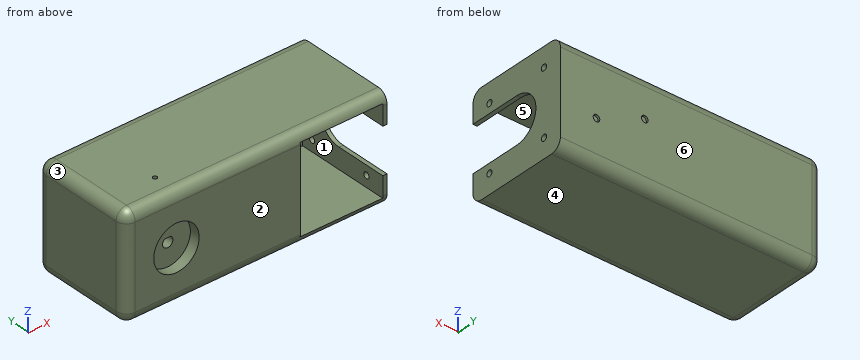
from build123d import *

# Parameters (mm, degrees)
F0_W           = 127
F0_H           = 50
F1_DEPTH       = 50
F3_DEPTH       = 42
F4_R           = 11
F5_DEPTH       = 5
F7_DEPTH       = 15
F8_T2_ANGLE    = 343.7894292622
F9_R           = 5
F12_W          = 40
F12_H          = 42
F13_DEPTH      = 46
F14_R          = 1.6
F15_DEPTH      = 1
F16_R          = 1
F17_DEPTH      = 2
F17_DEPTH_BACK = 1.03
F18_DEPTH      = 25
F19_DEPTH      = 2
F20_DEPTH      = 25


# Not quite as in the source:
# - a fillet or chamfer that OpenCascade refuses, or shapes differently, is made with other operations: its cross-section is extruded or revolved along the edge and cut away or added


with BuildPart() as f1:
    # F0 (on Front) → F1 (new body)
    with BuildSketch(Plane.XZ):
        Rectangle(F0_W, F0_H)
    extrude(amount=F1_DEPTH)

    # F2 (on face) → F3 (cut)
    with BuildSketch(Plane.YZ.offset(63.5)):
        Polygon((-41.7573593129, 21), (-46, 16.7573593129), (-46, -16.7573593129), (-41.7573593129, -21), (-8.2426406871, -21), (-4, -16.7573593129), (-4, 16.7573593129), (-8.2426406871, 21), align=None)
    extrude(amount=-F3_DEPTH, mode=Mode.SUBTRACT)

    # F4 (on face) → F5 (cut)
    with BuildSketch(Plane.XZ.offset(50)):
        with Locations((-38.5, 0)):
            Circle(F4_R)
    extrude(amount=-F5_DEPTH, mode=Mode.SUBTRACT)

    # F6 (on face) → F7 (cut)
    with BuildSketch(Plane.XZ.offset(45)):
        with BuildLine():
            Line((-37, 2), (-40, 2))
            ThreePointArc((-40, 2), (-38.5, -2.5), (-37, 2))
        make_face()
    extrude(amount=-F7_DEPTH, mode=Mode.SUBTRACT)

    # F8: fillet of radius 0.5 on 1 edges, made by hand

    # F8_s1 → F8_t2 (revolve)
    with BuildSketch(Plane(origin=(-37.7346622942, 0, -5.3739891953), x_dir=(0, 1, 0), z_dir=(0.9900106558, 0, 0.1409925581))):
        with BuildLine():
            ThreePointArc((-30.5, 7.9282134883), (-30.1464466094, 7.7817668789), (-30, 7.4282134883))
            Line((-30, 7.4282134883), (-30, 7.9282134883))
            Line((-30, 7.9282134883), (-30.5, 7.9282134883))
        make_face()
    revolve(axis=Axis((-38.5, -30, 0), (0, -1, 0)), revolution_arc=F8_T2_ANGLE)

    # F9
    f9_edges = [f1.edges().sort_by_distance(p)[0] for p in [
        (0, -50, 25),
        (0, -50, -25),
        (0, 0, 25),
        (0, 0, -25),
        (-63.5, -25, 25),
        (-63.5, -25, -25),
        (-63.5, 0, 0),
        (-63.5, -50, 0),
    ]]
    fillet(f9_edges, radius=F9_R)

    # F12 (on face) → F13 (cut)
    with BuildSketch(Plane.XZ.offset(50)):
        with Locations((41.5, 0)):
            Rectangle(F12_W, F12_H)
    extrude(amount=-F13_DEPTH, mode=Mode.SUBTRACT)

    # F14 (on face) → F15 (cut)
    with BuildSketch(Plane(origin=(0, 0, 0), x_dir=(-1, 0, 0), z_dir=(0, 1, 0))):
        with Locations((-46.0031795697, -4.1205275279)):
            Circle(F14_R)
        with Locations((-22.6282365388, 5.5031795697)):
            Circle(F14_R)
    extrude(amount=-F15_DEPTH, mode=Mode.SUBTRACT)

    # F16 (on face) → F17 (cut, two sides)
    with BuildSketch(Plane(origin=(0, 0, 2), x_dir=(1, 0, 0), z_dir=(0, 0, -1))) as f17_sk:
        Polygon((-36.5, 38.9047005384), (-38.5, 40.0594010768), (-40.5, 38.9047005384), (-40.5, 36.5952994616), (-38.5, 35.4405989232), (-36.5, 36.5952994616), align=None)
        with Locations((-38.5, 37.75)):
            Circle(F16_R, mode=Mode.SUBTRACT)
    extrude(amount=-F17_DEPTH, mode=Mode.SUBTRACT)
    extrude(f17_sk.sketch, amount=F17_DEPTH_BACK, mode=Mode.SUBTRACT)

    # F18 (cut): a face of the model
    f18_faces = [f1.faces().sort_by_distance(p)[0] for p in [
        (-38.5, -37.75, 2),
    ]]
    extrude(f18_faces, amount=-F18_DEPTH, mode=Mode.SUBTRACT)

    # F10 (on face) → F19 (join)
    with BuildSketch(Plane.YZ.offset(63.5)):
        Polygon((-46, 16.7573593129), (-46, -16.7573593129), (-41.7573593129, -21), (-8.2426406871, -21), (-4, -16.7573593129), (-4, 16.7573593129), (-8.2426406871, 21), (-16.9, 21), (-33.1, 21), (-41.7573593129, 21), align=None)
        with BuildLine():
            Line((-10.9, -15.6), (-39.1, -15.6))
            ThreePointArc((-39.1, -15.6), (-41.6606601718, -16.6606601718), (-40.6, -14.1))
            Line((-40.6, -14.1), (-40.6, 14.1))
            ThreePointArc((-40.6, 14.1), (-41.6606601718, 16.6606601718), (-39.1, 15.6))
            Line((-39.1, 15.6), (-10.9, 15.6))
            ThreePointArc((-10.9, 15.6), (-9.4, 17.1), (-7.9, 15.6))
            ThreePointArc((-7.9, 15.6), (-8.3393398282, 14.5393398282), (-9.4, 14.1))
            Line((-9.4, 14.1), (-9.4, -14.1))
            ThreePointArc((-9.4, -14.1), (-8.3393398282, -14.5393398282), (-7.9, -15.6))
            ThreePointArc((-7.9, -15.6), (-9.4, -17.1), (-10.9, -15.6))
        make_face(mode=Mode.SUBTRACT)
        with BuildLine():
            ThreePointArc((-40.6, -14.1), (-39.5393398282, -14.5393398282), (-39.1, -15.6))
            Line((-39.1, -15.6), (-10.9, -15.6))
            ThreePointArc((-10.9, -15.6), (-10.4606601718, -14.5393398282), (-9.4, -14.1))
            Line((-9.4, -14.1), (-9.4, 14.1))
            ThreePointArc((-9.4, 14.1), (-10.4606601718, 14.5393398282), (-10.9, 15.6))
            Line((-10.9, 15.6), (-39.1, 15.6))
            ThreePointArc((-39.1, 15.6), (-39.5393398282, 14.5393398282), (-40.6, 14.1))
            Line((-40.6, 14.1), (-40.6, -14.1))
        make_face()
    extrude(amount=-F19_DEPTH)

    # F11 (on face) → F20 (cut)
    with BuildSketch(Plane.YZ.offset(63.5)):
        with BuildLine():
            Line((-50, -11), (-25, -11))
            ThreePointArc((-25, -11), (-14, 0), (-25, 11))
            Line((-25, 11), (-50, 11))
            Line((-50, 11), (-50, -11))
        make_face()
    extrude(amount=-F20_DEPTH, mode=Mode.SUBTRACT)


solid = f1.part
Check sheet for the modelled part. Datum: model origin and axes. Units: mm. Face numbers are marked on the shaded views. A direction names the side the tool comes from. Give positions to 0.01 mm unless a question says otherwise; leave off trailing zeros. Loops run counter-clockwise (first coordinate to the right, second up) from the corner with the lowest first, then second, coordinate; pieces in that order, holes last. Notation, with made-up numbers: M 35,22 L 94,22 A23 cw 94,30 Z; hole C -29.5,22 d1. An arc over 180 degrees is marked long. Answer as a JSON object with one key per item and string values. Group by question number.
Q1. Material ranges on line 1 along X through (y, z) = (-32, -1.5); line 2 along X through (y, z) = (-7, 12.5); line 3 along Y through (x, z) = (62.7, -15.6), recorded low to high. Write a range as [from, to].
Q2. Cross-section at D-D on z = -9.5. Record the cut outline in (x, y), then the cut area to 3 significant figures.
Q3. Go/stop test with flat-tipped pins: P1, Ø1.8, axis at x = -38.5, y = -37.75, coming from the +Z side; P2, Ø17.5, axis at x = -38.5, z = 0, coming from the -Y side; P3, Ø1.9, axis at x = 46, z = -4.12, coming from the -Y side. Record where each tip stops, or that it passes through.
Q4. Release check for a two-part mould opening along Z. For the marked faces 1, 2, 3 and 4 record: released by +Z, released by -Z, zero draft, split by the parting line, or undercut.
Q5. Cross-section at A-A on x = 42. Record the cut outline in (y, z), then the cut area to 3 significant figures.
Q6. Cross-section at C-C on y = -20. Record the cut outline in (x, z).
Q7. Access from +Z, -Z, +X, -X, +Y, -Y to the whole of each face (thin tool, end or side, straight path). Record for the marked faces 5 and 6.
Q8. Cross-section at B-B on z = 0. Record the cut outline in (x, y).
Evaluation:
{
 "1": {"line 1": "x = [-63.5, -40.5], [-36.5, 21.5]", "line 2": "x = [-63.5, 21.5], [61.5, 63.5]", "line 3": "y = [-50, -42.1], [-39.1, -10.9], [-7.9, 0]"},
 "2": {"outline": "M -63.5,-45 A5 ccw -58.5,-50 L -44.05,-50 L -44.05,-45 L -32.95,-45 L -32.95,-50 L 21.5,-50 L 21.5,-4 L 61.5,-4 L 61.5,-19.45 L 63.5,-19.45 L 63.5,0 L -58.5,0 A5 ccw -63.5,-5 Z", "area": "4,380 mm2"},
 "3": {"P1": "stops at z = -2.33", "P2": "stops at y = -45", "P3": "stops at y = -4"},
 "4": {"face 1": "undercut", "face 2": "zero draft", "face 3": "released by +Z", "face 4": "released by -Z"},
 "5": {"outline": "M -49.9,-21 A5 ccw -45,-25 L -5,-25 A5 ccw 0,-20 L 0,20 A5 ccw -5,25 L -45,25 A5 ccw -49.9,21 L -4,21 L -4,-21 Z", "area": "547 mm2"},
 "6": {"outline": "M -63.5,-20 A5 ccw -58.5,-25 L 63.5,-25 L 63.5,-9.8 L 61.5,-9.8 L 61.5,-21 L 21.5,-21 L 21.5,21 L 61.5,21 L 61.5,9.8 L 63.5,9.8 L 63.5,25 L -58.5,25 A5 ccw -63.5,20 Z"},
 "7": {"face 5": "-Y", "face 6": "+Z, -Z, +X, -X, +Y"},
 "8": {"outline": "M -63.5,-45 A5 ccw -58.5,-50 L -49.5,-50 L -49.5,-45 L -41,-45 L -41,-30.5 A0.5 cw -40.5,-30 L -36.5,-30 A0.5 cw -36,-30.5 L -36,-45 L -27.5,-45 L -27.5,-50 L 21.5,-50 L 21.5,-4 L 61.5,-4 L 61.5,-14 L 63.5,-14 L 63.5,0 L -58.5,0 A5 ccw -63.5,-5 Z"}
}
